Source: three-view drawing plus pictorial views. Frame: mm from the lowest corner of the part. A direction names the side the tool comes from. Give positions to 0.01 mm unless a question says otherwise; leave off trailing zeros. Write each loop counter-clockwise with the first axis right and the second up, starting at its lowest first coordinate (ties: lowest second). Pieces come first, ordered by that corner, then holes. Notation, with made-up numbers: (89.5, 43.25) -> (145.5, 43.25) arc R27 cw to (145.5, 70.25) -> close; hole circle Ø1 at (-19.75, 39.25). An arc over 180 degrees is marked (long way). Answer in a Markdown table with one row per item. Add a question column.
Item 1: Section query B-B on y = 10. Output: boundary loops of the cut face in (x, z), plus the area to 3 significant figures.
Item 2: Section query D-D on x = 16.75. Output: boundary loops of the cut face in (y, z), plus the area to 3 significant figures.
Item 3: First-contact query: P1, Ø3, axis at y = 14.5, z = 17.5, coming from the -X side; P2, Ø10, axis at y = 22.5, z = 17, coming from the -X side; P3, Ø1, axis at x = 14.5, z = 10.5, coming from the +Y side. Flat tips, straight axial feed; report the tip coordinate or a pass-through.
Item 4: Material intervals for probe 1 along Y at (x, z) = (18.6, 10); probe 2 along Z at (x, y) = (19.25, 10); probe 3 along X at (y, z) = (1.3, 10), sorted ascending. Write a range as from..to.
Item 5: Section query A-A on x = 9. Output: boundary loops of the cut face in (y, z).
Item 6: Access query for the marked faces 5 and 6. Directions: +Z, -Z, +X, -X, +Y, -Y. A direction counts if a zero-diameter tool reaches every point of the face in a straight line with its end or side. Return the directions, or none.
Item 7: Section query C-C on z = 9.5. Output: boundary loops of the cut face in (x, y).
Item 8: Draft query along Z for the marked faces 1, 2, 3 and 4. Return one class per face: +Z half, -Z half, draft (parallel to the pull), parting line (faces both ways), or undercut.
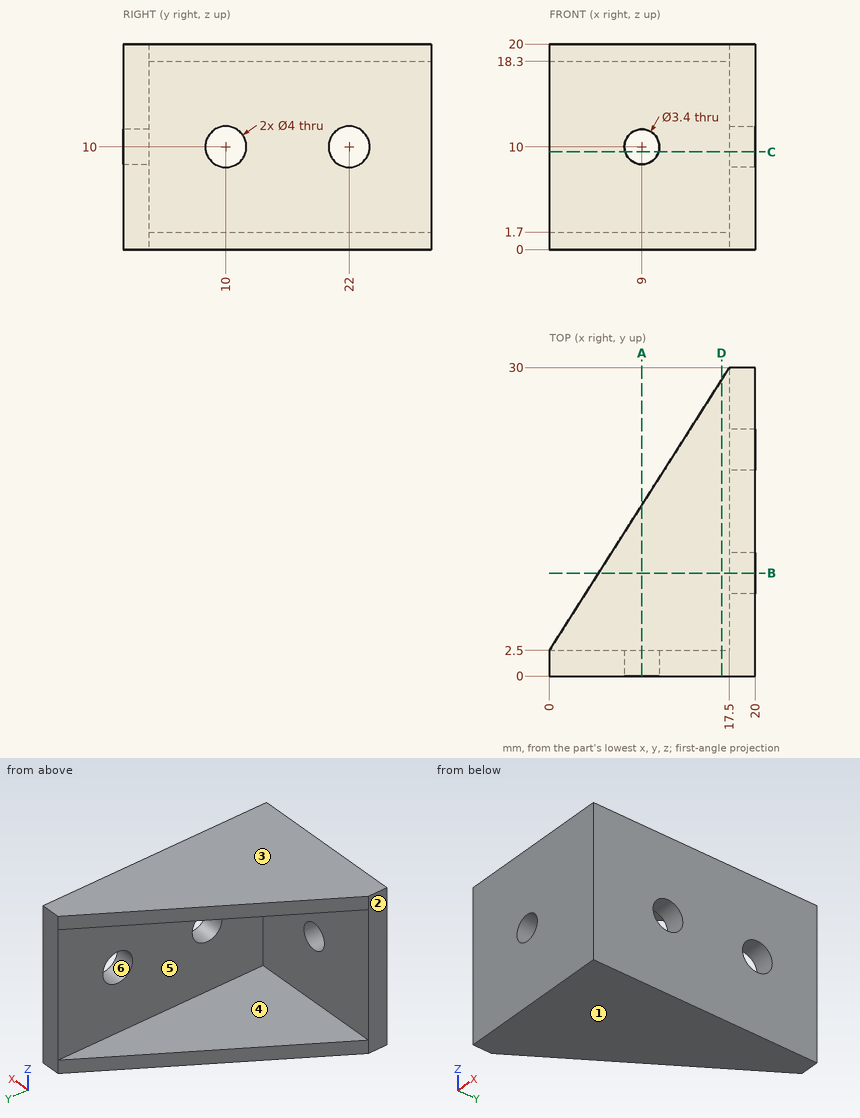
Findings below:
| question | item | result |
|---|---|---|
| 1 | outline | (4.77, 0) -> (20, 0) -> (20, 8) -> (17.5, 8) -> (17.5, 1.7) -> (4.77, 1.7) -> close; (4.77, 18.3) -> (17.5, 18.3) -> (17.5, 12) -> (20, 12) -> (20, 20) -> (4.77, 20) -> close |
| 1 | area | 83.3 mm^2 |
| 2 | outline | (0, 0) -> (28.82, 0) -> (28.82, 1.7) -> (2.5, 1.7) -> (2.5, 18.3) -> (28.82, 18.3) -> (28.82, 20) -> (0, 20) -> close |
| 2 | area | 139 mm^2 |
| 3 | P1 | stops at x = 6.83 |
| 3 | P2 | stops at x = 9.65 |
| 3 | P3 | stops at y = 2.5 |
| 4 | probe 1 | y = 0..8, 12..20, 24..30 |
| 4 | probe 2 | z = 0..8, 12..20 |
| 4 | probe 3 | x = 0..7.3, 10.7..20 |
| 5 | outline | (0, 0) -> (16.64, 0) -> (16.64, 1.7) -> (2.5, 1.7) -> (2.5, 8.3) -> (0, 8.3) -> close; (0, 11.7) -> (2.5, 11.7) -> (2.5, 18.3) -> (16.64, 18.3) -> (16.64, 20) -> (0, 20) -> close |
| 6 | face 5 | -X, +Y |
| 6 | face 6 | +X, -X |
| 7 | outline | (0, 0) -> (7.38, 0) -> (7.38, 2.5) -> (0, 2.5) -> close; (10.62, 0) -> (20, 0) -> (20, 8.06) -> (17.5, 8.06) -> (17.5, 2.5) -> (10.62, 2.5) -> close; (17.5, 11.94) -> (20, 11.94) -> (20, 20.06) -> (17.5, 20.06) -> close; (17.5, 23.94) -> (20, 23.94) -> (20, 30) -> (17.5, 30) -> close |
| 8 | face 1 | -Z half |
| 8 | face 2 | draft |
| 8 | face 3 | +Z half |
| 8 | face 4 | undercut |
